The model under review builds one solid part; all positions refer to its coordinate system, in mm. A direction names the side the tool comes from. Round coordinates to 2 decimals unless told otherwise and drop trailing zeros. Loops run counter-clockwise (first coordinate to the right, second up) from the corner with the lowest first, then second, coordinate; pieces in that order, holes last. Notation, with made-up numbers: M -24,17 L 26,17 A15 cw 26,39 Z; hole C 52.5,11.25 d1. An arc over 180 degrees is marked long. Answer as a JSON object with one key per item and string values. Group by question number.
Item 1: Consider section B-B (z = -480.5). Give the boundary of the cut face in (x, y).
Item 2: Consider section C-C (x = -421.5). Give the boundary of the cut face in (y, z).
Item 3: To check wall thickness, follow line 1 (Y direction, x = -313.5, z = -488.5); line 2 (Z direction, x = -365, y = 63); line 3 (X direction, y = 64.5, z = -155.5). State the ranges of each line that lie inside material, in increasing order.
Item 4: Consider section A-A (x = -354). Give the boundary of the cut face in (y, z).
Item 5: Insertion check: P1, Ø6, axis at x = -276.5, z = -147.5, coming from the +Y side; P2, Ø3, axis at x = -317.5, y = 393.5, coming from the -Z side. Each pin has a flat end and moves straight along its axis. Give the tip position at first contact, or say it passes through.
Item 6: Consider section D-D (z = -242). Give the boundary of the cut face in (x, y).
Item 7: The part is to be moulded in two halves that separate along Z. For faces 1 (the face through (-50, 49, -405)), 2 (the face through (-306.503, 603, -429.287)), 3 (the face through (-304, 54, -800)), 4 (the face through (-296, 54, 0)), say which applies: +Z half, -Z half, draft (parallel to the pull), parting line (faces both ways), or undercut.
Item 8: Tool access review of faces 5 (the face through (-379.357, 1119.86, -460.848)), 6 (the face through (-550, 49, -395)), 7 (the face through (-324, 1110, -379)), 8 (the face through (-600, 54, -394)): name each direction out of +Z, -Z, +X, -X, +Y, -Y from which nothing blocks a thin tool from reaching the whole face with its end or side.
Autodesk Inventor part; units mm, degrees
ref_plane "YZ Plane" through (0, 0, 0) normal (1, 0, 0) x (0, 1, 0)
ref_plane "XZ Plane" through (0, 0, 0) normal (0, 1, 0) x (-1, 0, 0)
ref_plane "XY Plane" through (0, 0, 0) normal (0, 0, 1) x (1, 0, 0)
sketch "Sketch1" plane through (0, 0, 0) normal (0, 1, 0) x (-1, 0, 0)
  line L0 (0, 0) -> (600, 0)
  line L1 (600, 0) -> (600, -800)
  line L2 (600, -800) -> (0, -800)
  line L3 (0, -800) -> (0, 0)
  line L4 (0, 0) -> (50, 0)
  line L5 (50, 0) -> (50, -50)
  line L6 (50, -50) -> (0, -50)
  line L7 (0, -50) -> (0, 0)
  line L8 (600, -800) -> (550, -800)
  line L9 (550, -800) -> (550, -750)
  line L10 (550, -750) -> (600, -750)
  line L11 (600, -750) -> (600, -800)
  line L12 (50, -50) -> (550, -50)
  line L13 (550, -50) -> (550, -750)
  line L14 (550, -750) -> (50, -750)
  line L15 (50, -750) -> (50, -50)
  dimension "d0" = 800
  dimension "d1" = 600
  dimension "d2" = 50
  dimension "d3" = 50
  dimension "d4" = 50
  dimension "d5" = 50
extrude "Extrusion1" add sketch "Sketch1" along normal blind 100 contours L0 L5 L6 L3 | L0 L1 L10 L13 L12 L5 | L6 L15 L14 L9 L2 L3 | L1 L2 L9 L10
sketch "Sketch2" plane through (0, 100, 0) normal (0, 1, 0) x (1, 0, 0)
  line L0 (-600, 800) -> (-600, 0)
  line L1 (0, 0) -> (0, 800)
  line L2 (-600, 0) -> (0, 0)
  line L3 (0, 0) -> (0, 800)
  line L4 (0, 800) -> (-600, 800)
  line L5 (-600, 800) -> (-600, 0)
  circle A0 centre (-300, 400) radius 25
  dimension "d8" = 50
extrude "Extrusion2" add sketch "Sketch2" along normal blind 10 contours L4 L1 L2 L0 | A0
sketch "Sketch3" plane through (0, 110, 0) normal (0, 1, 0) x (1, 0, 0)
  line L0 (0, 0) -> (0, 800)
  line L1 (0, 800) -> (-600, 800)
  line L2 (-600, 800) -> (-600, 0)
  line L3 (-600, 0) -> (0, 0)
  circle A0 centre (-300, 400) radius 30
  dimension "d11" = 60
extrude "Extrusion3" add sketch "Sketch3" along normal blind 1000 contours A0
sketch "Sketch4" plane through (-300, 1110, -400) normal (0, 1, 0) x (1, 0, 0)
  circle A0 centre (0, 0) radius 30
  circle A1 centre (0, 0) radius 100
  point P0 (300, -400)
  dimension "d14" = 200
extrude "Extrusion4" add sketch "Sketch4" along normal blind 20 contours A0 | A1
properties part number "Corte"
Geometry results:
{
 "1": {"outline": "M -600,0 L -550,0 L -550,100 L -50,100 L -50,0 L 0,0 L 0,110 L -600,110 Z; M -359.33,1110 L -240.67,1110 L -240.67,1130 L -359.33,1130 Z"},
 "2": {"outline": "M 0,-800 L 110,-800 L 110,0 L 0,0 L 0,-50 L 100,-50 L 100,-750 L 0,-750 Z"},
 "3": {"line 1": "y = 100 to 110, 1110 to 1130", "line 2": "z = -800 to -750, -50 to 0", "line 3": "x = -600 to -550, -50 to 0"},
 "4": {"outline": "M 0,-800 L 110,-800 L 110,0 L 0,0 L 0,-50 L 100,-50 L 100,-750 L 0,-750 Z; M 1110,-484.17 L 1130,-484.17 L 1130,-315.83 L 1110,-315.83 Z"},
 "5": {"P1": "stops at y = 110", "P2": "stops at z = -425.38"},
 "6": {"outline": "M -600,0 L -550,0 L -550,100 L -50,100 L -50,0 L 0,0 L 0,110 L -600,110 Z"},
 "7": {"face 1": "undercut", "face 2": "parting line", "face 3": "-Z half", "face 4": "+Z half"},
 "8": {"face 5": "+Y", "face 6": "-Y", "face 7": "none", "face 8": "+Z, -Z, -X, +Y, -Y"}
}
